The listing builds one solid part. Answer for the finished solid, in the listing's coordinates (mm). A direction names the side the tool comes from. Coordinates: 2 decimals unless noted, no trailing zeros. Order: outer loops, then holes, each group sorted by start corner. A loop starts at its lowest first (then second) coordinate and runs counter-clockwise, first axis right, second up.
```python
from build123d import *

# Parameters (mm, degrees)
F0_W      = 80
F0_H      = 41
F1_DEPTH  = 1.6
F3_DEPTH  = 8.24
F5_DEPTH  = 12.5
F7_DEPTH  = 7
F9_DEPTH  = 2
F11_DEPTH = 18.4
F12_R     = 0.5
F13_DEPTH = 7
F14_R     = 0.5
F15_DEPTH = 7
F16_R     = 0.5
F17_DEPTH = 7


with BuildPart() as f1:
    # F0 (on Top) → F1 (new body)
    with BuildSketch(Plane.XY):
        Rectangle(F0_W, F0_H)
    extrude(amount=F1_DEPTH)

    # F2 (on face) → F3 (join)
    with BuildSketch(Plane.XY.offset(1.6)):
        Polygon((40, -12.75), (40, 0), (40, 12.75), (33.5, 12.75), (33.5, -12.75), align=None)
        Polygon((40, 12.75), (40, 0), (40, -12.75), (45.5, -12.75), (45.5, 12.75), align=None)
    extrude(amount=F3_DEPTH)

    # F4 (on face) → F5 (join)
    with BuildSketch(Plane.XY.offset(1.6)):
        Polygon((-40, -15.5), (-40, 0), (-40, 15.5), (-43, 15.5), (-43, -15.5), align=None)
        Polygon((-40, 15.5), (-40, 0), (-40, -15.5), (-31, -15.5), (-31, 15.5), align=None)
    extrude(amount=F5_DEPTH)

    # F6 (on face) → F7 (join)
    with BuildSketch(Plane(origin=(-43, 0, 0), x_dir=(0, -1, 0), z_dir=(-1, 0, 0))):
        Polygon((0, 11.6), (0, 3.6), (5, 3.6), (8, 11.6), align=None)
        Polygon((-5, 3.6), (0, 3.6), (0, 11.6), (-8, 11.6), align=None)
        Polygon((-14, 10.448076), (-15.5, 7.85), (-14, 5.251924), (-11, 5.251924), (-9.5, 7.85), (-11, 10.448076), align=None)
        Polygon((15.098076, 9.35), (12.5, 10.85), (9.901924, 9.35), (9.901924, 6.35), (12.5, 4.85), (15.098076, 6.35), (15.098076, 7.85), align=None)
    extrude(amount=F7_DEPTH)

    # F8 (on face) → F9 (cut)
    with BuildSketch(Plane.XY.offset(1.6)):
        with BuildLine():
            ThreePointArc((37.7, 16.5), (37.26066, 17.56066), (36.2, 18))
            Line((36.2, 18), (36.2, 16.5))
            Line((36.2, 16.5), (36.2, 15))
            ThreePointArc((36.2, 15), (37.26066, 15.43934), (37.7, 16.5))
        make_face()
        with BuildLine():
            ThreePointArc((-23.3, -16.5), (-25.86066, -15.43934), (-24.8, -18))
            ThreePointArc((-24.8, -18), (-23.73934, -17.56066), (-23.3, -16.5))
        make_face()
        with BuildLine():
            ThreePointArc((37.7, -16.5), (37.26066, -15.43934), (36.2, -15))
            Line((36.2, -15), (36.2, -16.5))
            Line((36.2, -16.5), (36.2, -18))
            ThreePointArc((36.2, -18), (37.26066, -17.56066), (37.7, -16.5))
        make_face()
        with BuildLine():
            Line((36.2, -16.5), (36.2, -15))
            ThreePointArc((36.2, -15), (34.7, -16.5), (36.2, -18))
            Line((36.2, -18), (36.2, -16.5))
        make_face()
        with BuildLine():
            Line((36.2, 16.5), (36.2, 18))
            ThreePointArc((36.2, 18), (34.7, 16.5), (36.2, 15))
            Line((36.2, 15), (36.2, 16.5))
        make_face()
        with BuildLine():
            ThreePointArc((-24.8, 18), (-25.86066, 15.43934), (-23.3, 16.5))
            ThreePointArc((-23.3, 16.5), (-23.73934, 17.56066), (-24.8, 18))
        make_face()
    extrude(amount=-F9_DEPTH, mode=Mode.SUBTRACT)

    # F10 (on face) → F11 (join)
    with BuildSketch(Plane.XY.offset(1.6)):
        with BuildLine():
            ThreePointArc((-6, 15), (-6.732233, 16.767767), (-8.5, 17.5))
            Line((-8.5, 17.5), (-8.5, 15))
            Line((-8.5, 15), (-11, 15))
            ThreePointArc((-11, 15), (-8.5, 12.5), (-6, 15))
        make_face()
        with BuildLine():
            ThreePointArc((-12.6, -14.4), (-13.332233, -12.632233), (-15.1, -11.9))
            Line((-15.1, -11.9), (-15.1, -14.4))
            Line((-15.1, -14.4), (-15.1, -16.9))
            ThreePointArc((-15.1, -16.9), (-13.332233, -16.167767), (-12.6, -14.4))
        make_face()
        with BuildLine():
            Line((-15.1, -14.4), (-15.1, -11.9))
            ThreePointArc((-15.1, -11.9), (-17.6, -14.4), (-15.1, -16.9))
            Line((-15.1, -16.9), (-15.1, -14.4))
        make_face()
        with BuildLine():
            ThreePointArc((-15.1, 12.5), (-13.332233, 13.232233), (-12.6, 15))
            Line((-12.6, 15), (-15.1, 15))
            Line((-15.1, 15), (-15.1, 12.5))
        make_face()
        with BuildLine():
            Line((-15.1, 15), (-12.6, 15))
            ThreePointArc((-12.6, 15), (-16.867767, 16.767767), (-15.1, 12.5))
            Line((-15.1, 12.5), (-15.1, 15))
        make_face()
        with BuildLine():
            Line((-8.5, 15), (-8.5, 17.5))
            ThreePointArc((-8.5, 17.5), (-10.267767, 16.767767), (-11, 15))
            Line((-11, 15), (-8.5, 15))
        make_face()
    extrude(amount=F11_DEPTH)

    # F12 (on face) → F13 (join)
    with BuildSketch(Plane.XY.offset(20)):
        with Locations((-15.1, 15)):
            Circle(F12_R)
    extrude(amount=F13_DEPTH)

    # F14 (on face) → F15 (join)
    with BuildSketch(Plane.XY.offset(20)):
        with Locations((-8.5, 15)):
            Circle(F14_R)
    extrude(amount=F15_DEPTH)

    # F16 (on face) → F17 (join)
    with BuildSketch(Plane.XY.offset(20)):
        with Locations((-15.1, -14.4)):
            Circle(F16_R)
    extrude(amount=F17_DEPTH)


solid = f1.part
```
(1) Consider line 1 (X direction, y = 16.5, z = 0.45); line 2 (Y direction, x = -24.8, z = 0.7); line 3 (Z direction, x = 10.5, y = 14.5). Determine where each line is inside the solid, lowest interval first.
(2) Find section B-B (z = 23.25). Write down the section's boundary in (x, y).
(3) Find section D-D (x = -16.5). Write down the section's boundary in (y, z), and give its area (3 significant figures).
(4) Find section C-C (x = 15). Write down the section's boundary in (y, z), and give its area (3 significant figures).
(5) The mould has two halves that part along Y. Classify faces 6 (the face through (-37, 15.5, 8)), 7 (the face through (43, 0, 1.6)), 8 (the face through (-46.5, -11.2, 10.1)): released by +Y, released by -Y, zero draft, split by the parting line, or undercut.
(6) For faces 1 (the face through (-46.451, -6.479, 7.544)), 2 (the face through (-46, -9.902, 8)), 3 (the face through (-37, -15.5, 8)), 4 (the face through (-46.5, -13.8, 5.6)), 5 (the face through (-46, 13, 5.252)), determine the directions among +Z, -Z, +X, -X, +Y, -Y from which every point of the face is accessible in a straight line to the end or side of a thin tool.
(7) Find section A-A (z = 13). Write down the section's boundary in (x, y).
(8) Each of these flat-tipped pins is pushed along its axis until it touches: pin 1 Ø2.5 at (x, z) = (39.5, 7.5) entering from +Y; pin 2 Ø10 at (x, z) = (-12, 7.5) entering from +Y; pin 3 Ø2.5 at (x, z) = (-45.5, 8.5) entering from +Y; pin 4 Ø1.5 at (x, z) = (32.5, 12) entering from +Y. Where does it stop, or does it pass through?
Findings below:
1. line 1: x = -40 to -26.3, -23.3 to 34.7, 37.7 to 40
1. line 2: y = -20.5 to -18, -15 to 15, 18 to 20.5
1. line 3: z = 0 to 1.6
2. outline: circle Ø1 at (-15.1, -14.4); circle Ø1 at (-15.1, 15); circle Ø1 at (-8.5, 15)
3. outline: (-20.5, 0) - (20.5, 0) - (20.5, 1.6) - (17.07, 1.6) - (17.07, 20) - (12.93, 20) - (12.93, 1.6) - (-12.33, 1.6) - (-12.33, 20) - (-16.47, 20) - (-16.47, 1.6) - (-20.5, 1.6) - close
3. area: 218 mm2
4. outline: (-20.5, 0) - (20.5, 0) - (20.5, 1.6) - (-20.5, 1.6) - close
4. area: 65.6 mm2
5. face 6: released by +Y
5. face 7: zero draft
5. face 8: undercut
6. face 1: -Z, -X
6. face 2: +Z, -Z, -X
6. face 3: +Z, -X, -Y
6. face 4: -Z, -X, -Y
6. face 5: -Z, -X, +Y
7. outline: (-43, -15.5) - (-31, -15.5) - (-31, 15.5) - (-43, 15.5) - close; circle Ø5 at (-15.1, -14.4); circle Ø5 at (-15.1, 15); circle Ø5 at (-8.5, 15)
8. pin 1: stops at y = 12.75
8. pin 2: stops at y = 17.5
8. pin 3: stops at y = 15.5
8. pin 4: passes through
